```python
from build123d import *

# Parameters (mm, degrees)
SKETCH1_R           = 2
SKETCH1_R_2         = 20
BOSS_EXTRUDE1_DEPTH = 3
FILLET2_R           = 3
SKETCH2_R           = 22
SKETCH2_R_2         = 20
BOSS_EXTRUDE3_DEPTH = 10


with BuildPart() as part:
    # Sketch1 → Boss-Extrude1 (new body)
    with BuildSketch(Plane(origin=(0, 0, 0), x_dir=(1, 0, 0), z_dir=(0, 1, 0))):
        Polygon((0, 25), (-25, 25), (-25, -25), (25, -25), (25, 25), align=None)
        with Locations(Location((-19.091883092, 19.091883092, 0), (0, 0, 270))):
            Circle(SKETCH1_R, mode=Mode.SUBTRACT)
        with Locations(Location((19.091883092, 19.091883092, 0), (0, 0, 270))):
            Circle(SKETCH1_R, mode=Mode.SUBTRACT)
        with Locations(Location((19.091883092, -19.091883092, 0), (0, 0, 270))):
            Circle(SKETCH1_R, mode=Mode.SUBTRACT)
        with Locations(Location((-19.091883092, -19.091883092, 0), (0, 0, 270))):
            Circle(SKETCH1_R, mode=Mode.SUBTRACT)
        with Locations(Location((0, 0, 0), (0, 0, 270))):
            Circle(SKETCH1_R_2, mode=Mode.SUBTRACT)
    extrude(amount=BOSS_EXTRUDE1_DEPTH)

    # Fillet2
    fillet2_edges = [part.edges().sort_by_distance(p)[0] for p in [
        (25, 1.5, -25),
        (25, 1.5, 25),
        (-25, 1.5, 25),
        (-25, 1.5, -25),
    ]]
    fillet(fillet2_edges, radius=FILLET2_R)

    # Sketch2 → Boss-Extrude3 (add)
    with BuildSketch(Plane(origin=(0, 3, 0), x_dir=(1, 0, 0), z_dir=(0, 1, 0))):
        with Locations(Location((0, 0, 0), (0, 0, 270))):
            Circle(SKETCH2_R)
        with Locations(Location((0, 0, 0), (0, 0, 270))):
            Circle(SKETCH2_R_2, mode=Mode.SUBTRACT)
    extrude(amount=BOSS_EXTRUDE3_DEPTH)


solid = part.part
```
CAD build for the part. Positions are in the model's coordinates, mm. A direction names the side the tool comes from. Round coordinates to 2 decimals unless told otherwise and drop trailing zeros. Loops run counter-clockwise (first coordinate to the right, second up) from the corner with the lowest first, then second, coordinate; pieces in that order, holes last. Notation, with made-up numbers: M 27,-19 L 80,-19 A28 ccw 80,10 Z; hole C 53.5,77.25 d3. An arc over 180 degrees is marked long. Use a Markdown table: item, result. Add a question column.
(1) Cut at B-B (z = 0). Give the cut face in (x, y), and give its area (3 significant figures).
(2) Pull direction Z, two halves, no side cores. Call faces 3 (the face through (24.1, 1.52, 24.14)), 4 (the face through (24.1, 1.52, -24.14)), 5 (the face through (-18, 13, 10)), 6 (the face through (-19.524, 6.409, -4.336)): +Z half, -Z half, draft (parallel to the pull), parting line (faces both ways), or undercut.
(3) Which spindle directions (+Z, -Z, +X, -X, +Y, -Y) get a long thin tool onto all of the face, cutting with end or side? Do faces 1 (the face through (0, 1, 25)), 2 (the face through (-21.477, 7.93, -4.769)). Say none if no direction does.
(4) Drill centre lines: line 1 (X direction, y = 6, z = 0); line 2 (Y direction, x = -12, z = 22); line 3 (X direction, y = 2, z = 1). Where is each one in solid material? Low to high.
(5) Flat gauge pins, fed straight in: pin 1 (6 mm diameter, centred on y = 8, z = 4, fed in from +X); pin 2 (4 mm diameter, centred on x = 6.5, y = 7, fed in from -Z); pin 3 (6 mm diameter, centred on y = 9, z = -7, fed in from -X). Where does each tip first touch, or does it go through?
(6) Cut at C-C (y = 9.25). Give the cut face in (x, z), and give its area (3 significant figures).
(7) Cut at A-A (x = 0). Give the cut face in (y, z), and give its area (3 significant figures).
Geometry says:
| question | item | result |
|---|---|---|
| 1 | outline | M -25,0 L -20,0 L -20,13 L -22,13 L -22,3 L -25,3 Z; M 20,0 L 25,0 L 25,3 L 22,3 L 22,13 L 20,13 Z |
| 1 | area | 70.0 mm² |
| 2 | face 3 | +Z half |
| 2 | face 4 | -Z half |
| 2 | face 5 | draft |
| 2 | face 6 | undercut |
| 3 | face 1 | +Z, +X, -X, +Y, -Y |
| 3 | face 2 | +Y |
| 4 | line 1 | x = -22 to -20, 20 to 22 |
| 4 | line 2 | y = 0 to 3 |
| 4 | line 3 | x = -25 to -19.97, 19.97 to 25 |
| 5 | pin 1 | stops at x = 21.98 |
| 5 | pin 2 | stops at z = -21.53 |
| 5 | pin 3 | stops at x = -21.63 |
| 6 | outline | C 0,0 d44; hole C 0,0 d40 |
| 6 | area | 264 mm² |
| 7 | outline | M 0,-25 L 3,-25 L 3,-22 L 13,-22 L 13,-20 L 0,-20 Z; M 0,20 L 13,20 L 13,22 L 3,22 L 3,25 L 0,25 Z |
| 7 | area | 70.0 mm² |
